Study the drawing (mm; zero at the part's minimum x, y, z) and answer. A direction names the side the tool comes from. Give positions to 0.01 mm unless a question says otherwise; leave off trailing zeros. Write each loop counter-clockwise with the first axis right and the second up, starting at its lowest first coordinate (ties: lowest second). Pieces come first, ordered by that corner, then holes. Notation, with made-up numbers: (39.25, 32.5) - (98.25, 32.5) arc R27 ccw to (98.25, 58.5) - close; hole circle Ø4 at (-2, 60). An arc over 180 degrees is marked (long way). Return JSON: item names as keys, results as strings.
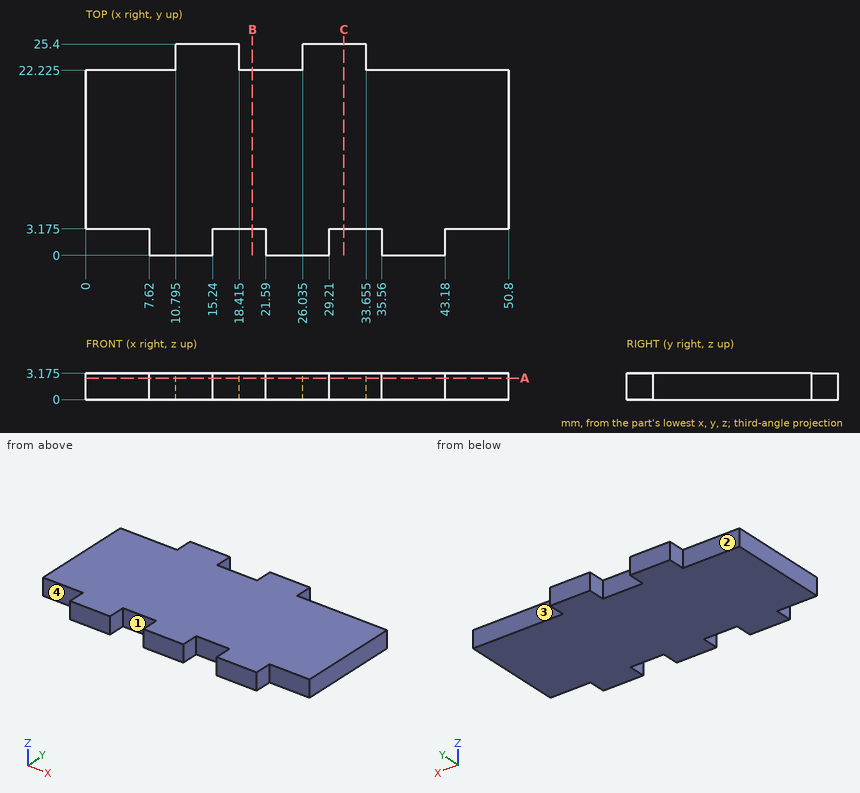
Item 1: Flat-ended cylindrical pins translate along their axes: P1, Ø1, axis at y = 1, z = 1, coming from the +X side; P2, Ø1, axis at y = 1.5, z = 2, coming from the -X side; P3, Ø1, axis at x = 2, z = 2, coming from the -Y side (3 decimals). Find the tip coordinate at first contact, or state that the pin passes through.
Answer below:
{"P1": "stops at x = 43.18", "P2": "stops at x = 7.62", "P3": "stops at y = 3.175"}
Item 2: Consider L1, parallel to Y at x = 23, z = 1.4 (3 decimals); L2, parallel to Y at x = 45.5, z = 2.95 (3 decimals). Determine where each line is inside the solid, lowest interval first.
Answer below:
{"L1": "y = 0 to 22.225", "L2": "y = 3.175 to 22.225"}
Item 3: A cutting plane is placed at C-C on x = 31. Determine the outline of the cut face in (y, z) (3 decimals), then the cut area to 3 significant figures.
Answer below:
{"outline": "(3.175, 0) - (25.4, 0) - (25.4, 3.175) - (3.175, 3.175) - close", "area": "70.6 mm²"}
Item 4: A cutting plane is placed at A-A on z = 2.6. Determine the outline of the cut face in (x, y) (3 decimals).
Answer below:
{"outline": "(0, 3.175) - (7.62, 3.175) - (7.62, 0) - (15.24, 0) - (15.24, 3.175) - (21.59, 3.175) - (21.59, 0) - (29.21, 0) - (29.21, 3.175) - (35.56, 3.175) - (35.56, 0) - (43.18, 0) - (43.18, 3.175) - (50.8, 3.175) - (50.8, 22.225) - (33.655, 22.225) - (33.655, 25.4) - (26.035, 25.4) - (26.035, 22.225) - (18.415, 22.225) - (18.415, 25.4) - (10.795, 25.4) - (10.795, 22.225) - (0, 22.225) - close"}
Item 5: For the marked faces 1, 2, 3 and 4, determine the directions among +Z, -Z, +X, -X, +Y, -Y from which every point of the face is accessible in a straight line to the end or side of a thin tool.
Answer below:
{"face 1": "+Z, -Z, -Y", "face 2": "+Z, -Z, -X, +Y", "face 3": "+Z, -Z, +X, +Y", "face 4": "+Z, -Z, -X, -Y"}
Item 6: A cutting plane is placed at B-B on x = 20. Determine the outline of the cut face in (y, z) (3 decimals).
Answer below:
{"outline": "(3.175, 0) - (22.225, 0) - (22.225, 3.175) - (3.175, 3.175) - close"}
